Model file for the job. Use its own axes, mm. Face numbers are marked on the shaded views. A direction names the side the tool comes from. Round coordinates to 2 decimals unless told otherwise and drop trailing zeros. Loops run counter-clockwise (first coordinate to the right, second up) from the corner with the lowest first, then second, coordinate; pieces in that order, holes last. Notation, with made-up numbers: (24, -10.75) - (44, -10.75) arc R25 cw to (44, 22.25) - close; hole circle Ø3 at (-9, -16.75). An arc over 180 degrees is marked (long way). Answer as a JSON object with one key per item and string values.
from build123d import *

# Parameters (mm, degrees)
F0_R     = 57.15
F0_R_2   = 0.9794958553
F1_DEPTH = 25.4
F3_T     = -7.62
F4_W     = 12.7
F4_H     = 33.02
F5_DEPTH = 25.4
F6_DEPTH = 25.4
F7_W     = 33.02
F7_H     = 6.35
F8_DEPTH = 25.4


# Not quite as in the source:
# - a feature of the source that left no trace in its solid (it failed there, or was rolled back) is left out


with BuildPart() as f1:
    # F0 (on Top) → F1 (new body)
    with BuildSketch(Plane.XY):
        Circle(F0_R)
        Circle(F0_R_2, mode=Mode.SUBTRACT)
    extrude(amount=F1_DEPTH)

    # F3
    f3_openings = [f1.faces().sort_by_distance(p)[0] for p in [
        (-57.15, 0, 12.7),
    ]]
    offset(amount=F3_T, openings=f3_openings)

    # F4 (on face) → F5 (cut)
    with BuildSketch(Plane.XY.offset(25.4)):
        with Locations((0, -28.575)):
            Rectangle(F4_W, F4_H)
    extrude(amount=-F5_DEPTH, mode=Mode.SUBTRACT)

    # F4 (on face) → F6 (cut)
    with BuildSketch(Plane.XY.offset(25.4)):
        with Locations((0, 28.575)):
            Rectangle(F4_W, F4_H)
        with Locations((0, -28.575)):
            Rectangle(F4_W, F4_H)
    extrude(amount=-F6_DEPTH, mode=Mode.SUBTRACT)

    # F7 (on face) → F8 (cut)
    with BuildSketch(Plane(origin=(0, 0, 0), x_dir=(1, 0, 0), z_dir=(0, 0, -1))):
        with Locations((28.575, 3.175)):
            Rectangle(F7_W, F7_H)
        with Locations((28.575, -3.175)):
            Rectangle(F7_W, F7_H)
        with Locations((-28.575, -3.175)):
            Rectangle(F7_W, F7_H)
        with Locations((-28.575, 3.175)):
            Rectangle(F7_W, F7_H)
    extrude(amount=-F8_DEPTH, mode=Mode.SUBTRACT)


solid = f1.part
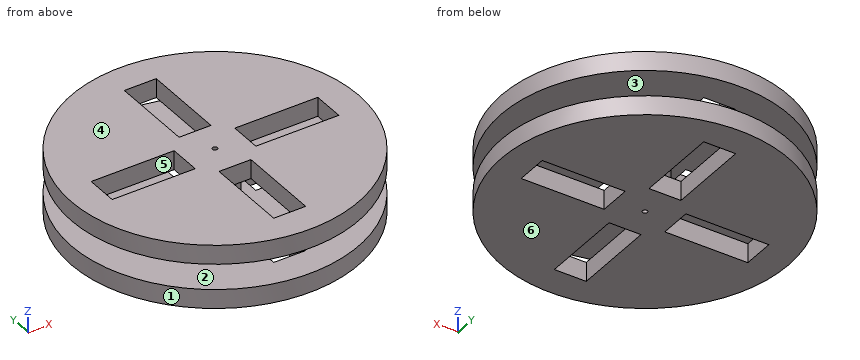
1) Probe probe 1 along X at (y, z) = (1.5, 21.75) (3 decimals); probe 2 along Y at (x, z) = (0, 17.25); probe 3 along Z at (x, y) = (-15.5, 21). List the from-to ranges inside material, lowest first.
Values follow:
{"probe 1": "-57.13 to -45.085, -12.065 to 12.065, 45.085 to 57.13", "probe 2": "-8.6 to -0.98, 0.98 to 8.6", "probe 3": "0 to 7.62, 17.78 to 25.4"}
2) Slice it at C-C on y = -23.5. List the corners of the cut face in (x, z), then the cut area to 3 significant figures.
Values follow:
{"outline": "(-52.09, 0) - (-6.35, 0) - (-6.35, 7.62) - (-52.09, 7.62) - close; (-52.09, 17.78) - (-6.35, 17.78) - (-6.35, 25.4) - (-52.09, 25.4) - close; (6.35, 0) - (52.09, 0) - (52.09, 7.62) - (6.35, 7.62) - close; (6.35, 17.78) - (52.09, 17.78) - (52.09, 25.4) - (6.35, 25.4) - close", "area": "1,390 mm²"}
3) Drop flat-ended pins along their axis: P1, Ø2.5, axis at y = -23, z = 2, coming from the +X side; P2, Ø2, axis at x = 2, z = 5, coming from the -Y side; P3, Ø2.5, axis at y = 32.5, z = 21.5, coming from the -X side. Give the stop position or say it passes through.
Values follow:
{"P1": "x = 52.85", "P2": "y = -57.14", "P3": "x = -47.85"}
4) Tool access for the marked faces 5 and 6: list every direction of +Z, -Z, +X, -X, +Y, -Y with a clear straight run to the whole face (end or side of a thin tool).
Values follow:
{"face 5": "+Z, -Z", "face 6": "-Z, +X, -X, +Y, -Y"}
5) Slice it at A-A on z = 2.5. Count the separate pieces of the cut face and the enclosed holes in it, then the cut area to 3 significant figures.
Values follow:
{"separate pieces": "1", "enclosed holes": "5", "area": "8,580 mm²"}
6) Slice it at B-B on x = -49.5. List the corners of the cut face in (y, z), then the cut area to 3 significant figures.
Values follow:
{"outline": "(-28.56, 0) - (28.56, 0) - (28.56, 7.62) - (-28.56, 7.62) - close; (-28.56, 17.78) - (28.56, 17.78) - (28.56, 25.4) - (-28.56, 25.4) - close", "area": "871 mm²"}
7) Slice it at D-D on y = -4. List the corners of the cut face in (x, z) (3 decimals).
Values follow:
{"outline": "(-57.01, 0) - (-45.085, 0) - (-45.085, 7.62) - (-57.01, 7.62) - close; (-57.01, 17.78) - (-45.085, 17.78) - (-45.085, 25.4) - (-57.01, 25.4) - close; (-12.065, 0) - (12.065, 0) - (12.065, 7.62) - (7.613, 7.62) - (7.613, 17.78) - (12.065, 17.78) - (12.065, 25.4) - (-12.065, 25.4) - (-12.065, 17.78) - (-7.613, 17.78) - (-7.613, 7.62) - (-12.065, 7.62) - close; (45.085, 0) - (57.01, 0) - (57.01, 7.62) - (45.085, 7.62) - close; (45.085, 17.78) - (57.01, 17.78) - (57.01, 25.4) - (45.085, 25.4) - close"}
8) Two-plate mould, pull along Z, no slides. Class the marked faces 1, 2, 3 and 4: pulls with the +Z half, pulls with the -Z half, needs draft (parallel to the pull), parting line crosses it, or undercut.
Values follow:
{"face 1": "needs draft", "face 2": "undercut", "face 3": "undercut", "face 4": "pulls with the +Z half"}
